Read the model definition and answer for the solid it produces. Units are mm, in the model's axes. A direction names the side the tool comes from. Coordinates: 2 decimals unless noted, no trailing zeros. Write each loop counter-clockwise with the first axis right and the second up, starting at its lowest first coordinate (ties: lowest second). Pieces come first, ordered by that corner, then holes. Notation, with made-up numbers: (48.5, -22) -> (97.5, -22) arc R14 ccw to (97.5, -18) -> close; hole circle Ø4 at (34.5, 85.25). An arc over 180 degrees is marked (long way). One line per item, written item: value. Start each with the question number.
1. Given P1, Ø5, axis at x = 7, y = 13.5, coming from the +Z side; P2, Ø6.5, axis at x = 10, y = 15.5, coming from the -Z side; P3, Ø0.5, axis at y = 20, z = 7, coming from the -X side; P4, Ø8, axis at x = 6.5, z = -1, coming from the -Y side, each flat-ended and moving along its own axis, determine where each tip first touches the part or whether it passes through.
2. Find section A-A, the plane z = 0. Write down the section's boundary in (x, y).
3. For a pull along X with two mould halves and no side action, classify faces 6 (the flat face through (8, 10, -29)), 7 (the flat face through (10.741, 24.919, -32.803)), 8 (the flat face through (16, 22, 0)) as pulls with the +X half, pulls with the -X half, needs draft (parallel to the pull), parting line crosses it, or undercut.
4. Find section B-B, the plane z = 17. Write down the section's boundary in (x, y), and give its area (3 significant figures).
5. Find section C-C, the plane z = -15.5. Write down the section's boundary in (x, y).
6. For faces 1 (the flat face through (3.5, 20, 0)), 2 (the flat face through (2, 19, 5.7)), 3 (the flat face through (8, 25, 34.4)), 4 (the flat face through (8, 0, 27)), 5 (the flat face through (8, 14, 26.25)), determine the directions among +Z, -Z, +X, -X, +Y, -Y from which every point of the face is accessible in a straight line to the end or side of a thin tool.
7. Consider line 1 along Z through (x, y) = (2.5, 16.5); line 2 along Z through (x, y) = (8, 5); line 3 along X through (y, z) = (15.75, 15). Determine where each line is inside the solid, lowest interval first.
```python
from build123d import *

# Parameters (mm, degrees)
SKETCH001_W     = 23.25
SKETCH001_H     = 46.5
POCKET_DEPTH    = 16.001
POCKET001_DEPTH = 21
SKETCH003_W     = 4.5
SKETCH003_H     = 1
GROOVE_ANGLE    = 65
SKETCH004_W     = 6
SKETCH004_H     = 1
GROOVE001_ANGLE = 7
PAD_DEPTH       = 16
SKETCH006_W     = 8
SKETCH006_H     = 10
POCKET002_DEPTH = 16.001
SKETCH007_R     = 1.6
POCKET003_DEPTH = 26.251
POCKET004_DEPTH = 2.7
FILLET_R        = 7.999
SKETCH009_R     = 1.6
POCKET005_DEPTH = 16.001


with BuildPart() as part:
    # Sketch → Revolution (revolve)
    with BuildSketch(Plane.XY):
        Polygon((0, -18.5), (10, -18.5), (10, -21.25), (14.5, -21.25), (14.5, -20.05), (16, -20.05), (16, -23.25), (14.5, -23.25), (10, -23.25), (0, -23.25), align=None)
    revolve(axis=Axis((0, 0, 0), (1, 0, 0)))

    # Sketch001 (on Face9 of Revolution) → Pocket (cut, through all)
    with BuildSketch(Plane.YZ.offset(16)):
        with Locations((-11.625, 0)):
            Rectangle(SKETCH001_W, SKETCH001_H)
    extrude(amount=-POCKET_DEPTH, mode=Mode.SUBTRACT)

    # Sketch002 (on Face2 of Pocket) → Pocket001 (cut)
    with BuildSketch(Plane.XZ):
        Polygon((0, 8.5), (10, 8.5), (10, 5.7), (6.3, 5.7), (6.3, -5.7), (10, -5.7), (10, -8.5), (0, -8.5), (0, -5.7), (3.5, -5.7), (3.5, 5.7), (0, 5.7), align=None)
    extrude(amount=-POCKET001_DEPTH, mode=Mode.SUBTRACT)

    # Sketch003 (on Face4 of Pocket001) → Groove (revolve, cut)
    with BuildSketch(Plane.XZ):
        with Locations((12.25, -21.75)):
            Rectangle(SKETCH003_W, SKETCH003_H)
    groove = revolve(axis=Axis((0, 0, 0), (1, 0, 0)), revolution_arc=GROOVE_ANGLE, mode=Mode.SUBTRACT)

    # Sketch004 (on Face4 of Groove) → Groove001 (revolve, cut)
    with BuildSketch(Plane.XZ):
        with Locations((12.25, -21.75)):
            Rectangle(SKETCH004_W, SKETCH004_H)
    groove001 = revolve(axis=Axis((0, 0, 0), (1, 0, 0)), revolution_arc=GROOVE001_ANGLE, mode=Mode.SUBTRACT)

    # Sketch005 (on Face12 of Groove001) → Pad (join)
    with BuildSketch(Plane(origin=(0, 0, 0), x_dir=(0, -1, 0), z_dir=(-1, 0, 0))):
        with BuildLine():
            ThreePointArc((0, 23.25), (-23.25, 0), (0, -23.25))
            Line((0, -36.25), (0, -23.25))
            Line((-26.25, -36.25), (0, -36.25))
            Line((-26.25, -36.25), (-26.25, 36.25))
            Line((-26.25, 36.25), (0, 36.25))
            Line((0, 36.25), (0, 23.25))
        make_face()
    extrude(amount=-PAD_DEPTH)

    # Sketch006 (on Face11 of Pad) → Pocket002 (cut, through all)
    with BuildSketch(Plane.YZ.offset(16)):
        with Locations((14, 31.25)):
            Rectangle(SKETCH006_W, SKETCH006_H)
        with Locations((14, -31.25)):
            Rectangle(SKETCH006_W, SKETCH006_H)
    extrude(amount=-POCKET002_DEPTH, mode=Mode.SUBTRACT)

    # Sketch007 (on Face40 of Pocket002) → Pocket003 (cut, through all)
    with BuildSketch(Plane(origin=(0, 26.25, 0), x_dir=(-1, 0, 0), z_dir=(0, 1, 0))):
        with Locations((-8, 31.25)):
            Circle(SKETCH007_R)
        with Locations((-8, -31.25)):
            Circle(SKETCH007_R)
    extrude(amount=-POCKET003_DEPTH, mode=Mode.SUBTRACT)

    # Sketch008 (on Face41 of Pocket003) → Pocket004 (cut)
    with BuildSketch(Plane(origin=(0, 26.25, 0), x_dir=(-1, 0, 0), z_dir=(0, 1, 0))):
        Polygon((-9.818653, 34.4), (-11.637307, 31.25), (-9.818653, 28.1), (-6.181347, 28.1), (-4.362693, 31.25), (-6.181347, 34.4), align=None)
        Polygon((-9.818653, -28.1), (-11.637307, -31.25), (-9.818653, -34.4), (-6.181347, -34.4), (-4.362693, -31.25), (-6.181347, -28.1), align=None)
    extrude(amount=-POCKET004_DEPTH, mode=Mode.SUBTRACT)

    # Mirrored: Groove001, Groove across XY
    add(groove001.mirror(Plane.XY), mode=Mode.SUBTRACT)
    add(groove.mirror(Plane.XY), mode=Mode.SUBTRACT)

    # Fillet
    fillet_edges = [part.edges().sort_by_distance(p)[0] for p in [
        (0, 22.125, 36.25),
        (0, 5, 36.25),
        (16, 5, 36.25),
        (16, 22.125, 36.25),
        (0, 22.125, -36.25),
        (0, 5, -36.25),
        (16, 22.125, -36.25),
        (16, 5, -36.25),
    ]]
    fillet(fillet_edges, radius=FILLET_R)

    # Sketch009 (on Face7 of Fillet) → Pocket005 (cut, through all)
    with BuildSketch(Plane.YZ.offset(16)):
        with Locations((20.007097, 22.008097)):
            Circle(SKETCH009_R)
        with Locations((20.007097, -22.008097)):
            Circle(SKETCH009_R)
    extrude(amount=-POCKET005_DEPTH, mode=Mode.SUBTRACT)


solid = part.part
```
Answer block:
1. P1: stops at z = 26.25
1. P2: stops at z = -36.25
1. P3: stops at x = 10
1. P4: stops at y = 17.81
2. outline: (0, 18.5) -> (3.5, 18.5) -> (3.5, 21) -> (6.3, 21) -> (6.3, 18.5) -> (10, 18.5) -> (10, 21.25) -> (14.5, 21.25) -> (14.5, 20.05) -> (16, 20.05) -> (16, 26.25) -> (0, 26.25) -> close
3. face 6: needs draft
3. face 7: undercut
3. face 8: pulls with the +X half
4. outline: (0, 7.3) -> (10, 7.3) -> (10, 14.35) -> (14.5, 14.35) -> (14.5, 10.63) -> (16, 10.63) -> (16, 26.25) -> (0, 26.25) -> close
4. area: 266 mm2
5. outline: (0, 10.1) -> (10, 10.1) -> (10, 15.96) -> (14.5, 15.96) -> (14.5, 12.72) -> (16, 12.72) -> (16, 26.25) -> (0, 26.25) -> close
6. face 1: -Y
6. face 2: -X, -Y
6. face 3: +Y
6. face 4: +Z, -Z, +X, -X, -Y
6. face 5: +Z, +X, -X
7. line 1: z = -26.25 to -8.5, 8.5 to 26.25
7. line 2: z = -36.25 to -32.85, -29.65 to -17.81, 17.81 to 29.65, 32.85 to 36.25
7. line 3: x = 0 to 10, 14.5 to 16
